The model under review builds one solid part; all positions refer to its coordinate system, in mm. Face numbers are marked on the shaded views. A direction names the side the tool comes from. Round coordinates to 2 decimals unless told otherwise and drop trailing zeros. Write each loop counter-clockwise with the first axis right and the second up, starting at its lowest first coordinate (ties: lowest second). Pieces come first, ordered by that corner, then holes. Notation, with made-up numbers: M 65,-12.5 L 124,-12.5 A9 ccw 124,-3.5 Z; hole C -15,75.25 d6. An arc over 180 degrees is marked long. Write item = value, one per line. Start each with the question number.
Item 1: Tool access review of the marked faces 1, 2 and 3: name each direction out of +Z, -Z, +X, -X, +Y, -Y from which nothing blocks a thin tool from reaching the whole face with its end or side.
Item 2: Take a section at B-B, the plane x = -11.25. Give the boundary of the cut face in (y, z) (3 decimals), plus the area to 3 significant figures.
Item 3: To check wall thickness, follow line 1 along Z through (x, y) = (-13.75, 0) (3 decimals); line 2 along Y through (x, z) = (2.5, -1.25) (3 decimals). State the ranges of each line that lie inside material, in increasing order.
Item 4: Take a section at D-D, the plane x = -0.5. Give the boundary of the cut face in (y, z) (3 decimals).
Item 5: For pin 1 Ø1 at (x, z) = (-6.5, -0.5) entering from -Y, flat-tipped, find the tip position at first contact; note if it passes through.
Item 6: Take a section at C-C, the plane y = 4. Give the boundary of the cut face in (x, z) (1 decimal), plus the area to 3 significant figures.
Item 7: The part is to be moulded in two halves that separate along Z. For the marked faces 4, 5 and 6, say which applies: +Z half, -Z half, draft (parallel to the pull), parting line (faces both ways), or undercut.
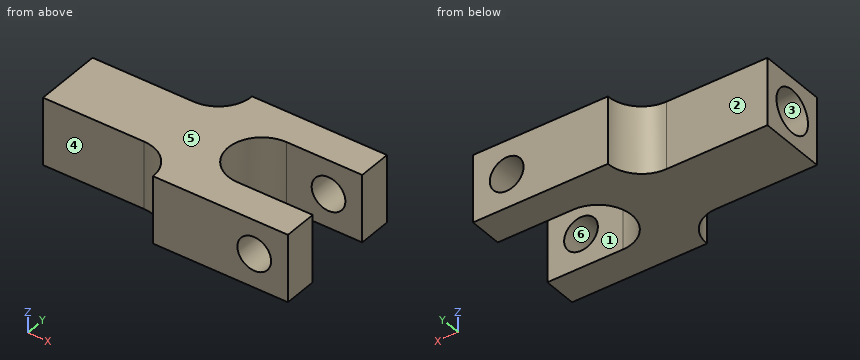
from build123d import *

# Parameters (mm, degrees)
F1_DEPTH = 3.175
F2_R     = 3.17499
F4_D     = 3.175
F6_D     = 4.0386
F6_DEPTH = 13.462
F6_TIP   = 1.213317848


# Not quite as in the source:
# - a fillet or chamfer is up to 0.001 mm smaller than in the source, because OpenCascade refuses the exact size


with BuildPart() as f1:
    # F0 (on Top) → F1 (new body, symmetric)
    with BuildSketch(Plane.XY):
        with BuildLine():
            Line((-5.588, -3.175), (-5.588, -6.35))
            Line((-5.588, -6.35), (7.112, -6.35))
            Line((7.112, -6.35), (7.112, -3.175))
            Line((7.112, -3.175), (0, -3.175))
            ThreePointArc((0, -3.175), (-3.175, 0), (0, 3.175))
            Line((0, 3.175), (7.112, 3.175))
            Line((7.112, 3.175), (7.112, 6.35))
            Line((7.112, 6.35), (-5.588, 6.35))
            Line((-5.588, 6.35), (-5.588, 3.175))
            Line((-5.588, 3.175), (-18.288, 3.175))
            Line((-18.288, 3.175), (-18.288, -3.175))
            Line((-18.288, -3.175), (-5.588, -3.175))
        make_face()
    extrude(amount=F1_DEPTH, both=True)

    # F2 (radius 3.175 in the source; OpenCascade refuses exactly that, so slightly less here)
    f2_edges = [f1.edges().sort_by_distance(p)[0] for p in [
        (-5.588, -3.175, 0),
        (-5.588, 3.175, 0),
    ]]
    fillet(f2_edges, radius=F2_R)

    # F4 (through all)
    with Locations(Plane.XZ.offset(6.35)):
        with Locations((3.937, 0)):
            Hole(F4_D / 2)

    # F6
    with Locations(Plane(origin=(-18.288, 0, 0), x_dir=(0, -1, 0), z_dir=(-1, 0, 0))):
        with Locations((0, 0)):
            Hole(F6_D / 2, depth=F6_DEPTH)
            with Locations((0, 0, -(F6_DEPTH + F6_TIP / 2))):  # 118° drill point
                Cone(0, F6_D / 2, F6_TIP, mode=Mode.SUBTRACT)


solid = f1.part
Response values:
q1.face_1 = +Z, -Z, +X
q1.face_2 = +Z, -Z, -X, +Y
q1.face_3 = -X
q2.outline = M -3.175,-3.175 L 3.175,-3.175 L 3.175,3.175 L -3.175,3.175 Z; hole C 0,0 d4.039
q2.area = 27.5 mm2
q3.line_1 = -3.175 to -2.019, 2.019 to 3.175
q3.line_2 = -6.35 to -3.175, 3.175 to 6.35
q4.outline = M -6.35,-3.175 L -3.135,-3.175 L -3.135,3.175 L -6.35,3.175 Z; M 3.135,-3.175 L 6.35,-3.175 L 6.35,3.175 L 3.135,3.175 Z
q5.pin_1 = -4.79
q6.outline = M -6.6,-3.2 L 7.1,-3.2 L 7.1,3.2 L -6.6,3.2 Z; hole C 3.9,0 d3.2
q6.area = 79.3 mm2
q7.face_4 = draft
q7.face_5 = +Z half
q7.face_6 = undercut
